```python
from build123d import *

# Parameters (mm, degrees)
SKETCH_1_W     = 30
SKETCH_1_H     = 4.75
CHAMFER_1_SIZE = 1
CHAMFER_2_SIZE = 1


with BuildPart() as part:
    # Эскиз1 → Повернуть1 (revolve)
    with BuildSketch(Plane.XY, mode=Mode.PRIVATE) as revolve_1_sk:
        with Locations((15, 17.625)):
            Rectangle(SKETCH_1_W, SKETCH_1_H)
    revolve(revolve_1_sk.sketch.rotate(Axis((0, 0, 0), (-1, 0, 0)), 90), axis=Axis((0, 0, 0), (-1, 0, 0)))

    # Фаска1
    chamfer_1_edges = [part.edges().sort_by_distance(p)[0] for p in [
        (0, 0, 20),
        (30, 0, 20),
    ]]
    chamfer(chamfer_1_edges, length=CHAMFER_1_SIZE)

    # Фаска2
    chamfer_2_edges = [part.edges().sort_by_distance(p)[0] for p in [
        (30, 0, 15.25),
        (0, 0, 15.25),
    ]]
    chamfer(chamfer_2_edges, length=CHAMFER_2_SIZE)


solid = part.part
```
Check sheet for the modelled part. Datum: model origin and axes. Units: mm. Round coordinates to 2 decimals unless told otherwise and drop trailing zeros. Loops run counter-clockwise (first coordinate to the right, second up) from the corner with the lowest first, then second, coordinate; pieces in that order, holes last. Notation, with made-up numbers: (67, 66) -> (111, 66) arc R17 ccw to (111, 72) -> close; hole circle Ø10 at (7, -15.75). An arc over 180 degrees is marked (long way). Answer in a Markdown table with one row per item.
Q1. Sectioned sample at A-A on z = 0. Enter the section's corners in (x, y).
Data:
| item | result |
|---|---|
| outline | (0, -19) -> (1, -20) -> (29, -20) -> (30, -19) -> (30, -16.25) -> (29, -15.25) -> (1, -15.25) -> (0, -16.25) -> close; (0, 16.25) -> (1, 15.25) -> (29, 15.25) -> (30, 16.25) -> (30, 19) -> (29, 20) -> (1, 20) -> (0, 19) -> close |
Q2. Thickness scan on L1, parallel to Y at x = 20.5, z = 0; L2, parallel to Z at x = 10.25, y = -9.5; L3, parallel to Y at x = 20.75, z = 14. Record the ranges inside material, lowest first.
Data:
| item | result |
|---|---|
| L1 | y = -20 to -15.25, 15.25 to 20 |
| L2 | z = -17.6 to -11.93, 11.93 to 17.6 |
| L3 | y = -14.28 to -6.05, 6.05 to 14.28 |
Q3. Sectioned sample at C-C on x = 28. Enter the section's corners in (y, z), then the cut area to 3 significant figures.
Data:
| item | result |
|---|---|
| outline | circle Ø40 at (0, 0); hole circle Ø30.5 at (0, 0) |
| area | 526 mm^2 |
Q4. Release check for a two-part mould opening along Y. For faces 1 (the face through (15.2, -0.88, 19.98)), 2 (the face through (15.196, 14.887, 3.306)), 3 (the face through (0, -9, 14)) record: released by +Y, released by -Y, zero draft, split by the parting line, or undercut.
Data:
| item | result |
|---|---|
| face 1 | split by the parting line |
| face 2 | undercut |
| face 3 | zero draft |
Q5. Go/stop test with flat-tipped pins: P1, Ø1, axis at y = -13.5, z = -7, coming from the +X side; P2, Ø10, axis at x = 13.5, z = 3.5, coming from the -Y side; P3, Ø4, axis at x = 20, y = 8, coming from the -Z side. Record where each tip stops, or that it passes through.
Data:
| item | result |
|---|---|
| P1 | stops at x = 29.46 |
| P2 | stops at y = -20 |
| P3 | stops at z = -19.08 |
